Part model, mm, in its own coordinate system. A direction names the side the tool comes from. Coordinates: 2 decimals unless noted, no trailing zeros. Loops run counter-clockwise (first coordinate to the right, second up) from the corner with the lowest first, then second, coordinate; pieces in that order, holes last. Notation, with made-up numbers: (-15.5, -29.75) - (-0.5, -29.75) arc R10 ccw to (-0.5, -12.75) - close; hole circle Ø1 at (48, -21.5). An arc over 180 degrees is marked (long way). Use a Markdown table: item, result. Add a question column.
1. Band-saw the part on A-A, the plane x = -7.5. Give the cut face in (y, z).
2. Wall check: probe 1 along Y at (x, z) = (18, -29.5); probe 2 along X at (y, z) = (-26, 1.5); probe 3 along X at (y, z) = (-33.5, -13.5). Give the ranges that are in metal, low to high. Write a range as [from, to].
3. Band-saw the part on C-C, the plane z = -11. Give the cut face in (x, y), plus the area to 3 significant figures.
4. Band-saw the part on D-D, the plane x = -24. Give the cut face in (y, z), plus the area to 3 significant figures.
5. 3-axis set-ups, long thin cutter, end or side, ignore diameter. For faces 1 (the flat face through (0, 3, 28)), 2 (the flat face through (-45, 3, 31.57)), 3 (the flat face through (-59, 0, 28)): which of +Z, -Z, +X, -X, +Y, -Y reach the whole face in a straight line?
6. Band-saw the part on B-B, the plane y = -22. Give the cut face in (x, z), plus the area to 3 significant figures.
7. Drop flat-ended pins along their axis: pin 1 (10 mm diameter, centred on y = -10, z = -5.5, fed in from -X); pin 2 (2 mm diameter, centred on x = -25.5, y = -6.5, fed in from +Z); pin 3 (10 mm diameter, centred on y = -44, z = 28.5, fed in from +X). Give the stop position or say it passes through.
from build123d import *

# Parameters (mm, degrees)
F0_R     = 42.6143864145
F0_R_2   = 6.7521330408
F1_DEPTH = 25.4
F2_DEPTH = 25.4
F3_W     = 89.4087702036
F3_H     = 6.2658451498
F4_DEPTH = 5.334


with BuildPart() as f1:
    # F0 (on Front) → F1 (new body)
    with BuildSketch(Plane.XZ):
        Circle(F0_R)
        Circle(F0_R_2, mode=Mode.SUBTRACT)
        Circle(F0_R_2)
    extrude(amount=F1_DEPTH)

    # F2 (add): a face of the model
    f2_faces = [f1.faces().sort_by_distance(p)[0] for p in [
        (0, -25.4, 0),
    ]]
    extrude(f2_faces, amount=F2_DEPTH)

    # F3 (on Front) → F4 (join)
    with BuildSketch(Plane.XZ):
        with Locations((-44.7043851018, 28.437288478)):
            Rectangle(F3_W, F3_H)
    extrude(amount=-F4_DEPTH)


solid = f1.part
Geometry check:
| question | item | result |
|---|---|---|
| 1 | outline | (-50.8, -41.95) - (0, -41.95) - (0, 25.3) - (5.33, 25.3) - (5.33, 31.57) - (0, 31.57) - (0, 41.95) - (-50.8, 41.95) - close |
| 2 | probe 1 | y = [-50.8, 0] |
| 2 | probe 2 | x = [-42.59, 42.59] |
| 2 | probe 3 | x = [-40.42, 40.42] |
| 3 | outline | (-41.17, -50.8) - (41.17, -50.8) - (41.17, 0) - (-41.17, 0) - close |
| 3 | area | 4,180 mm^2 |
| 4 | outline | (-50.8, -35.21) - (0, -35.21) - (0, 25.3) - (5.33, 25.3) - (5.33, 31.57) - (0, 31.57) - (0, 35.21) - (-50.8, 35.21) - close |
| 4 | area | 3,610 mm^2 |
| 5 | face 1 | +Z, -Z, +X, +Y |
| 5 | face 2 | +Z, +X, -X, +Y |
| 5 | face 3 | +Z, -X, -Y |
| 6 | outline | circle Ø85.23 at (0, 0) |
| 6 | area | 5,710 mm^2 |
| 7 | pin 1 | stops at x = -42.61 |
| 7 | pin 2 | stops at z = 34.87 |
| 7 | pin 3 | stops at x = 35.55 |
